Could you check a few things on this model? Use its own coordinates, in mm. A direction names the side the tool comes from. Coordinates: 2 decimals unless noted, no trailing zeros. Return JSON: item names as keys, results as strings. Group by question number.
from build123d import *

# Parameters (mm, degrees)
BOSS_EXTRUDE1_DEPTH = 68.2
SKETCH2_W           = 72.2
SKETCH2_H           = 15
BOSS_EXTRUDE2_DEPTH = 2
SKETCH3_W           = 72.2
SKETCH3_H           = 15
BOSS_EXTRUDE3_DEPTH = 2


with BuildPart() as part:
    # Sketch1 → Boss-Extrude1 (new body)
    with BuildSketch(Plane(origin=(0, 0, 0), x_dir=(0, 0, -1), z_dir=(1, 0, 0))):
        with BuildLine():
            Line((0, 0), (72.2, 0))
            add(Edge.make_bspline(
                [(0, 50.5), (16.749312519, 1.14415236), (72.2, 0)],
                knots=[0, 0, 0, 1, 1, 1], degree=2))
            Line((0, 50.5), (0, 0))
        make_face()
    extrude(amount=BOSS_EXTRUDE1_DEPTH)

    # Sketch2 → Boss-Extrude2 (add)
    with BuildSketch(Plane.ZY):
        with Locations((-36.1, 7.5)):
            Rectangle(SKETCH2_W, SKETCH2_H)
    extrude(amount=BOSS_EXTRUDE2_DEPTH)

    # Sketch3 → Boss-Extrude3 (add)
    with BuildSketch(Plane(origin=(68.2, 0, 0), x_dir=(0, 0, -1), z_dir=(1, 0, 0))):
        with Locations((36.1, 7.5)):
            Rectangle(SKETCH3_W, SKETCH3_H)
    extrude(amount=BOSS_EXTRUDE3_DEPTH)


solid = part.part
(1) Will these pins go through, and if not, where does the flat tip stop? P1, Ø12, axis at x = 29, y = 36, coming from the -Z side; P2, Ø1, axis at x = -1, z = -49, coming from the +Y side; P3, Ø3, axis at x = 24.5, z = -9.5, coming from the +Y side; P4, Ø5, axis at y = 15.5, z = -26.5, coming from the -X side.
(2) For faces 1 (the face through (68.2, 25, -6)), 2 (the face through (-1, 15, -37)), 3 (the face through (0, 9, -54)), which set-ups out of +Z, -Z, +X, -X, +Y, -Y let a thin tool reach every point of the face, with its end or its side?
(3) If I drill on L1, parallel to X at y = 20, z = -10.5; L2, parallel to X at y = 13, z = -54.5; L3, parallel to Y at x = 38, z = -36, over which ranges is the centre line in solid material (lowest first)? Write a range as [from, to].
Checks:
{
 "1": {"P1": "z = -9.99", "P2": "y = 15", "P3": "y = 33.09", "P4": "x = -2"},
 "2": {"face 1": "+Z, -Z, +X, +Y", "face 2": "+Z, -Z, -X, +Y", "face 3": "-Z, +Y"},
 "3": {"L1": "[0, 68.2]", "L2": "[-2, 0], [68.2, 70.2]", "L3": "[0, 7.66]"}
}
